Can you work these out from the drawing? Everything is in mm from the part's minimum corner. Round coordinates to 2 decimals unless told otherwise and drop trailing zeros. Write each loop counter-clockwise with the first axis right and the second up, starting at its lowest first coordinate (ties: lowest second). Pieces come first, ordered by that corner, then holes. Notation, with made-up numbers: M -11.5,-23 L 25.5,-23 A33 ccw 25.5,12 Z; hole C 18,80.5 d1. An arc over 180 degrees is marked long. Answer in a Markdown table with one row per item. Add a question column.
(1) I'm going to push flat-ended pins straight in: pin 1 (4 mm diameter, centred on x = 2.5, y = 218, fed in from +Z) (1 decimal); pin 2 (1 mm diameter, centred on y = 62, z = 3.5, fed in from -X); pin 3 (2 mm diameter, centred on x = 1.5, z = 13, fed in from +Y); pin 4 (4 mm diameter, centred on x = 2, y = 218.5, fed in from -Z). Where does each tip first touch, or does it pass through?
(2) If I drill on probe 1 along Z at (x, y) = (7.25, 123.5) (1 decimal); probe 2 along Y at (x, z) = (1.25, 2.75) (1 decimal); probe 3 along Y at (x, z) = (0.5, 4) (1 decimal), over which ranges is the centre line in solid material (lowest first)?
(3) Suppose I cut it at B-B, the plane y = 142.5. Write out the boundary of the cut face in (x, z) (1 decimal).
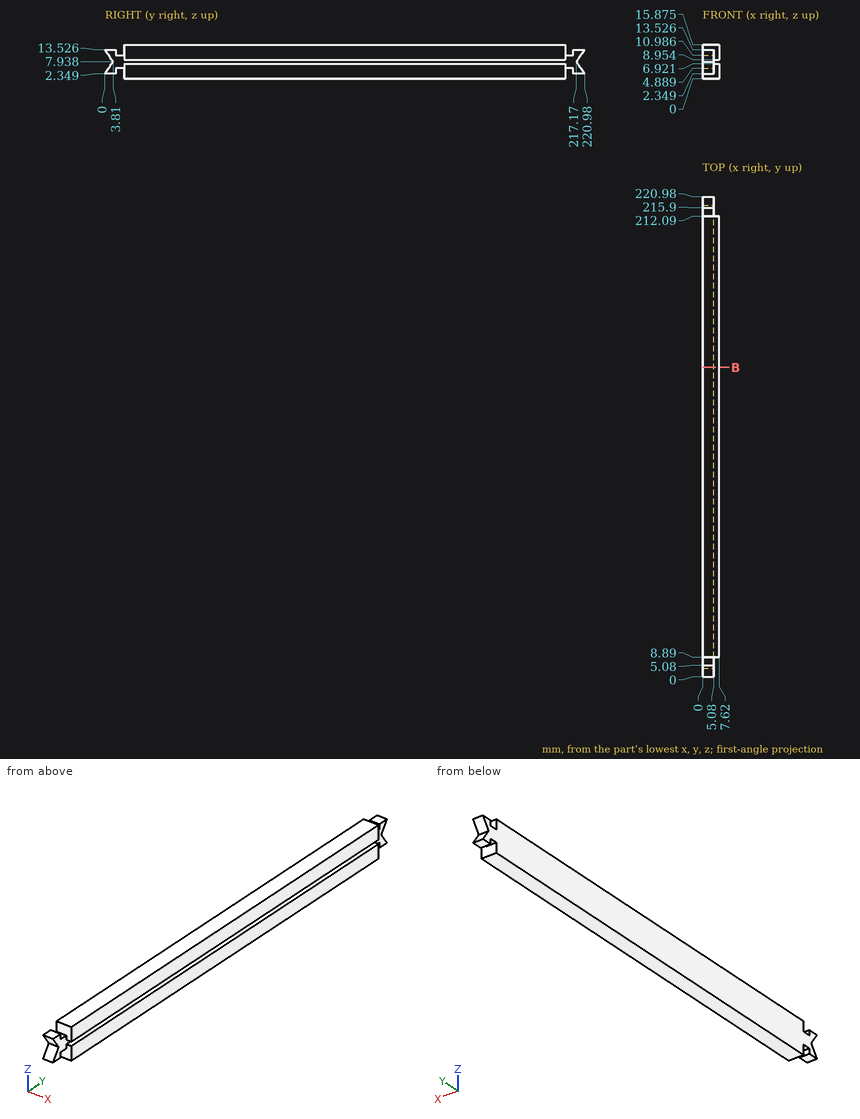
Calculated:
| question | item | result |
|---|---|---|
| 1 | pin 1 | z = 13.5 |
| 1 | pin 2 | x = 0 |
| 1 | pin 3 | y = 220.98 |
| 1 | pin 4 | z = 2.35 |
| 2 | probe 1 | 0 to 6.9, 9 to 15.9 |
| 2 | probe 2 | 0.3 to 5.1, 8.9 to 212.1, 215.9 to 220.7 |
| 2 | probe 3 | 1.1 to 5.1, 8.9 to 212.1, 215.9 to 219.9 |
| 3 | outline | M 0,0 L 7.6,0 L 7.6,6.9 L 5.1,6.9 L 5.1,9 L 7.6,9 L 7.6,15.9 L 0,15.9 Z |
